```python
from build123d import *

# Parameters (mm, degrees)
SKETCH_1_W          = 100
SKETCH_1_H          = 18
EXTRUDE_1_DEPTH     = 1
CHAMFER_1_SIZE      = 1
SKETCH_3_R          = 1.5
CUT_EXTRUDE_2_DEPTH = 20


with BuildPart() as part:
    # Эскиз1 → Бобышка-Вытянуть1 (new body)
    with BuildSketch(Plane(origin=(0, 0, 0), x_dir=(1, 0, 0), z_dir=(0, 1, 0))):
        Rectangle(SKETCH_1_W, SKETCH_1_H)
    extrude(amount=EXTRUDE_1_DEPTH)

    # Фаска1
    chamfer_1_edges = [part.edges().sort_by_distance(p)[0] for p in [
        (0, 1, 9),
    ]]
    chamfer(chamfer_1_edges, length=CHAMFER_1_SIZE - 0.0001)  # a hair under: the kernel refuses the full size

    # Эскиз3 → Вырез-Вытянуть2 (cut)
    with BuildSketch(Plane(origin=(0, 1, 0), x_dir=(1, 0, 0), z_dir=(0, 1, 0))):
        with Locations(Location((-43.709679881, 0.5, 0), (0, 0, 270))):
            Circle(SKETCH_3_R)
        with Locations(Location((43.709679881, 0.5, 0), (0, 0, 90))):
            Circle(SKETCH_3_R)
    extrude(amount=-CUT_EXTRUDE_2_DEPTH, mode=Mode.SUBTRACT)


solid = part.part
```
Check sheet for the modelled part. Datum: model origin and axes. Units: mm. Give positions to 0.01 mm unless a question says otherwise; leave off trailing zeros. Write each loop counter-clockwise with the first axis right and the second up, starting at its lowest first coordinate (ties: lowest second). Pieces come first, ordered by that corner, then holes. Notation, with made-up numbers: (4, 36.25) - (15, 36.25) arc R33 ccw to (15, 71.25) - close; hole circle Ø11 at (74, -26). An arc over 180 degrees is marked (long way). Answer as a JSON object with one key per item and string values. Group by question number.
1) Depth check by flat-ended pin: P1, Ø4, axis at x = -43.71, z = -0.5, coming from the -Y side. Enter the tip coordinate at first touch or a pass-through.
2) Thickness scan on probe 1 along X at (y, z) = (0.2, -0.5); probe 2 along X at (y, z) = (0.7, -1.75); probe 3 along Z at (x, y) = (-43, 0.9). Record the ranges inside material, lowest first. Write a range as from..to.
3) Sectioned sample at B-B (y = 0.2). Record the cut outline in (x, z), then the cut area to 3 significant figures.
4) Sectioned sample at A-A (z = -0.5). Record the cut outline in (x, y).
5) Release check for a two-part mould opening along Z. For faces 1 (the face through (-42.7, 0.51, -1.61)), 2 (the face through (-1, 0, 0)) record: pulls with the +Z half, pulls with the -Z half, needs draft (parallel to the pull), parting line crosses it, or undercut.
Geometry results:
{
 "1": {"P1": "stops at y = 0"},
 "2": {"probe 1": "x = -50..-45.21, -42.21..42.21, 45.21..50", "probe 2": "x = -50..-44.54, -42.88..42.88, 44.54..50", "probe 3": "z = -9..-1.82, 0.82..8.1"},
 "3": {"outline": "(-50, -9) - (50, -9) - (50, 8.8) - (-50, 8.8) - close; hole circle Ø3 at (-43.71, -0.5); hole circle Ø3 at (43.71, -0.5)", "area": "1,770 mm^2"},
 "4": {"outline": "(-50, 0) - (-45.21, 0) - (-45.21, 1) - (-50, 1) - close; (-42.21, 0) - (42.21, 0) - (42.21, 1) - (-42.21, 1) - close; (45.21, 0) - (50, 0) - (50, 1) - (45.21, 1) - close"},
 "5": {"face 1": "undercut", "face 2": "needs draft"}
}
